Verification items for the finished model (mm, model axes). A direction names the side the tool comes from. Give positions to 0.01 mm unless a question says otherwise; leave off trailing zeros. Order: outer loops, then holes, each group sorted by start corner. A loop starts at its lowest first (then second) coordinate and runs counter-clockwise, first axis right, second up. Notation, with made-up numbers: (60.25, 16.5) - (68.25, 16.5) arc R15 ccw to (68.25, 41.5) - close; hole circle Ø2 at (33, 78.25). An arc over 180 degrees is marked (long way). Answer as a JSON object with one key per item and string values.
```python
from build123d import *

# Parameters (mm, degrees)
SKETCH1_R               = 22.5
BOSS_EXTRUDE1_DEPTH     = 5
CUT_EXTRUDE1_DEPTH      = 4
CUT_EXTRUDE6_DEPTH      = 33.210246817
CUT_EXTRUDE6_DEPTH_BACK = 33.210246817
CUT_EXTRUDE7_START      = -1
SKETCH5_R               = 1.5
CUT_EXTRUDE7_DEPTH      = 1
CRVPATTERN3_COUNT       = 10


with BuildPart() as part:
    # Sketch1 → Boss-Extrude1 (new body)
    with BuildSketch(Plane(origin=(0, 0, 0), x_dir=(1, 0, 0), z_dir=(0, 1, 0))):
        with Locations(Location((0, 0, 0), (0, 0, 270))):
            Circle(SKETCH1_R)
    extrude(amount=BOSS_EXTRUDE1_DEPTH)

    # Sketch2 → Cut-Extrude1 (cut)
    with BuildSketch(Plane(origin=(0, 5, 0), x_dir=(1, 0, 0), z_dir=(0, 1, 0))):
        with BuildLine():
            Line((-1.160818677, -0.95), (1.160818677, -0.95))
            ThreePointArc((1.160818677, -0.95), (0, 1.5), (-1.160818677, -0.95))
        make_face()
    extrude(amount=-CUT_EXTRUDE1_DEPTH, mode=Mode.SUBTRACT)

    # Sketch4 → Cut-Extrude6 (cut, two sides: drawn at the far end of the back side and taken through both)
    with BuildSketch(Plane(origin=(0, 5, 0), x_dir=(1, 0, 0), z_dir=(0, 1, 0)).offset(-CUT_EXTRUDE6_DEPTH_BACK)):
        Polygon((83.285175452, 104.034655768), (-2.447970935, 22.36643553), (-7.154384821, 17.883170165), (-13.654384821, 17.883170165), (-132.059919263, 17.883170165), (-220.021178565, 237.751992892), (-4.67608385, 323.903478495), align=None)
    cut_extrude6 = extrude(amount=CUT_EXTRUDE6_DEPTH + CUT_EXTRUDE6_DEPTH_BACK, mode=Mode.SUBTRACT)

    # Sketch5 → Cut-Extrude7 (cut)
    with BuildSketch(Plane.XZ.offset(CUT_EXTRUDE7_START)):
        with Locations(Location((0, 0, 0), (0, 0, 39.296480239))):
            Circle(SKETCH5_R)
    extrude(amount=CUT_EXTRUDE7_DEPTH, mode=Mode.SUBTRACT)

    # CrvPattern3: Cut-Extrude6 ×10 about axis
    crvpattern3_axis = Axis((0, 0, 0), (0, -1, 0))
    for i in range(1, CRVPATTERN3_COUNT):
        add(cut_extrude6.rotate(crvpattern3_axis, i * 360 / CRVPATTERN3_COUNT), mode=Mode.SUBTRACT)


solid = part.part
```
(1) Section check D-D (z = -15). Record the cut outline in (x, y).
Computed values:
{"outline": "(-15.43, 0) - (13.93, 0) - (13.93, 5) - (-15.43, 5) - close"}
(2) Gauge pin test, flat ends, axial feed: pin 1 Ø1.5 at (x, y) = (-10, 3.5) entering from -Z; pin 2 Ø1 at (y, z) = (4.5, -13) entering from -X; pin 3 Ø1.5 at (y, z) = (1, 13) entering from -X. Record the tip position at first contact, or that the pin passes through.
Computed values:
{"pin 1": "stops at z = -17.88", "pin 2": "stops at x = -15.89", "pin 3": "stops at x = -14.95"}
(3) Access from +Z, -Z, +X, -X, +Y, -Y to the whole of each face (thin tool, end or side, straight path). Record for faces 1 (the flat face through (-10, 2, -17.883)), 2 (the flat face through (0, 3, 0.95)), 3 (the flat face through (2.06, 2.46, -20.61)).
Computed values:
{"face 1": "-Z, -X, +Y, -Y", "face 2": "+Y, -Y", "face 3": "-Z, +Y, -Y"}
(4) Release check for a two-part mould opening along X. For faces 4 (the flat face through (7.99, 2.46, -19.11)), 5 (the cylindrical face through (21.81, 2.46, 5.53)), 6 (the cylindrical face through (-21.81, 2.46, -5.53)) record: pulls with the +X half, pulls with the -X half, needs draft (parallel to the pull), parting line crosses it, or undercut.
Computed values:
{"face 4": "undercut", "face 5": "pulls with the +X half", "face 6": "pulls with the -X half"}
(5) Material ranges on line 1 along Z through (x, y) = (0, 0.35); line 2 along X through (y, z) = (0.3, 0); line 3 along Z through (x, y) = (0, 3.2), recorded low to high. Write a range as [from, to].
Computed values:
{"line 1": "z = [-22.1, -1.5], [1.5, 22.1]", "line 2": "x = [-19.83, -1.5], [1.5, 19.83]", "line 3": "z = [-22.1, -1.5], [0.95, 22.1]"}
(6) Section check C-C (z = 0). Record the cut outline in (x, y).
Computed values:
{"outline": "(-19.83, 0) - (-1.5, 0) - (-1.5, 5) - (-19.83, 5) - close; (1.5, 0) - (19.83, 0) - (19.83, 5) - (1.5, 5) - close"}
(7) Section check B-B (x = 0). Record the cut outline in (y, z).
Computed values:
{"outline": "(0, -22.1) - (5, -22.1) - (5, -1.5) - (0, -1.5) - close; (0, 1.5) - (1, 1.5) - (1, 0.95) - (5, 0.95) - (5, 22.1) - (0, 22.1) - close"}
